Job drawing, mm, ordinate dimensions from the low corner. One solid piece. A direction names the side the tool comes from. Give positions to 0.01 mm unless a question says otherwise; leave off trailing zeros. Write each loop counter-clockwise with the first axis right and the second up, starting at its lowest first coordinate (ties: lowest second). Pieces come first, ordered by that corner, then holes. Notation, with made-up numbers: (65.25, -10.75) -> (116.25, -10.75) arc R30 cw to (116.25, 24.25) -> close; hole circle Ø1 at (-24.75, 35). An arc over 180 degrees is marked (long way). Put each result on its own line as item: value. Start each with the question number.
Item 1: Slice it at A-A, the plane y = 50. List the corners of the cut face in (x, z), plus the area to 3 significant figures.
Item 2: Slice it at D-D, the plane x = 24.5. List the corners of the cut face in (y, z).
Item 3: Flat gauge pins, fed straight in: pin 1 Ø4 at (y, z) = (56.5, 171) entering from +X; pin 2 Ø6 at (x, y) = (43, 85) entering from +Z; pin 3 Ø5 at (y, z) = (50.5, 218.5) entering from -X. Where does each tip first touch, or does it go through?
Item 4: Slice it at C-C, the plane z = 150. List the corners of the cut face in (x, y).
Item 5: Tool access for the marked faces 1 and 2: list every direction of +Z, -Z, +X, -X, +Y, -Y with a clear straight run to the whole face (end or side of a thin tool).
Item 6: Drill centre lines: line 1 along Z through (x, y) = (43, 29); line 2 along Z through (x, y) = (4, 22); line 3 along X through (y, z) = (51.5, 120). Where is each one in solid material? Low to high.
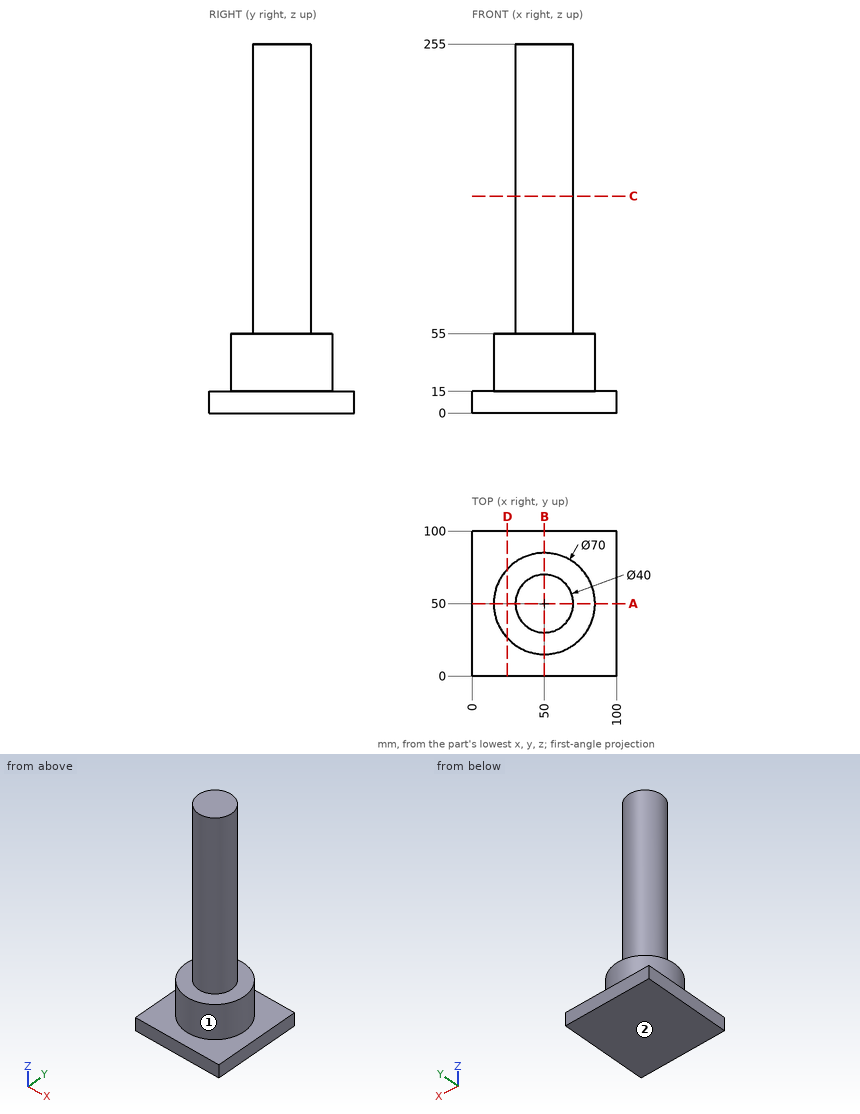
Values follow:
1. outline: (0, 0) -> (100, 0) -> (100, 15) -> (85, 15) -> (85, 55) -> (70, 55) -> (70, 255) -> (30, 255) -> (30, 55) -> (15, 55) -> (15, 15) -> (0, 15) -> close
1. area: 12,300 mm2
2. outline: (0, 0) -> (100, 0) -> (100, 15) -> (73.97, 15) -> (73.97, 55) -> (26.03, 55) -> (26.03, 15) -> (0, 15) -> close
3. pin 1: x = 69.49
3. pin 2: z = 55
3. pin 3: x = 30
4. outline: circle Ø40 at (50, 50)
5. face 1: +Z
5. face 2: -Z, +X, -X, +Y, -Y
6. line 1: 0 to 55
6. line 2: 0 to 15
6. line 3: 30.06 to 69.94
